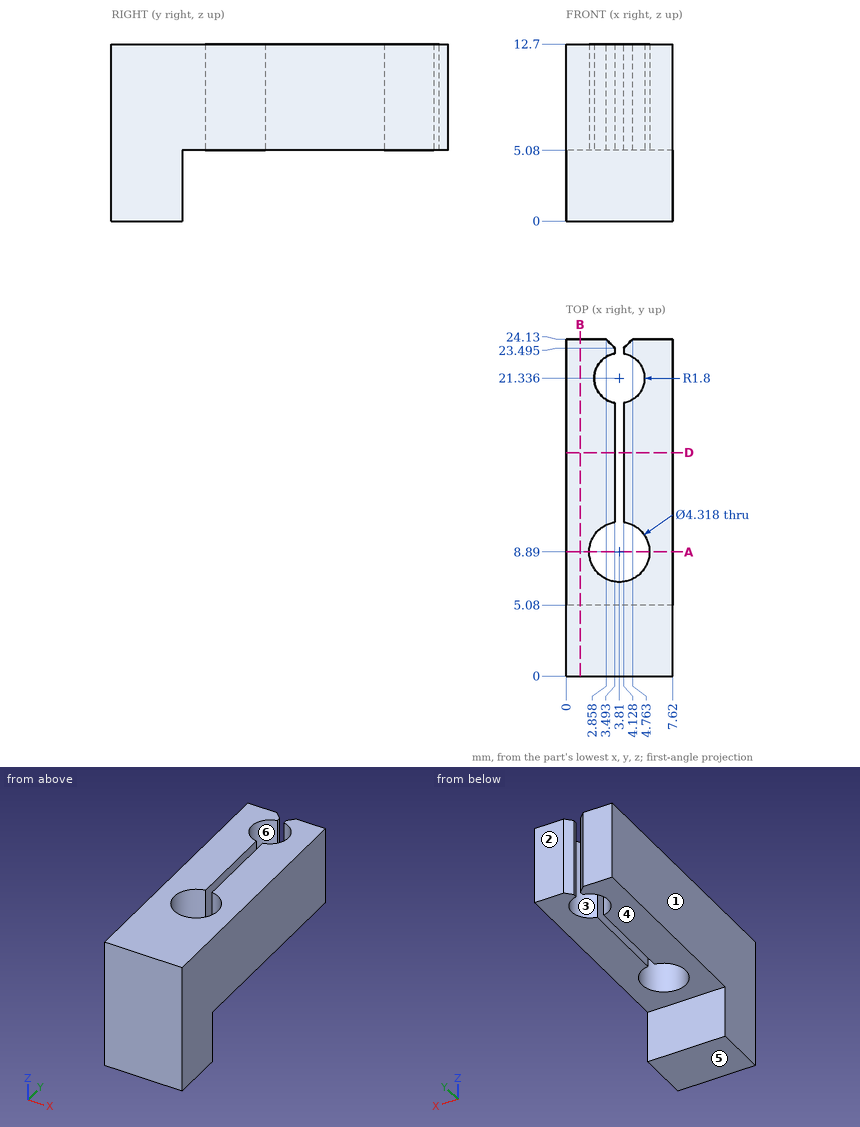
Answer from the drawing. Dimensions are ordinates in mm from the lowest x, y and z of the part. A direction names the side the tool comes from. Coordinates: 2 decimals unless noted, no trailing zeros. Write each loop counter-clockwise with the first axis right and the second up, starting at its lowest first coordinate (ties: lowest second). Pieces come first, ordered by that corner, then holes. Notation, with made-up numbers: (20, 73) - (43, 73) arc R11 cw to (43, 87) - close; hole circle Ø9 at (83, 59). An arc over 180 degrees is marked (long way). One line per question, with ' | ' between items.
Q1. Consider L1, parallel to X at y = 8.89, z = 7; L2, parallel to Y at x = 2.75, z = 10; L3, parallel to X at y = 14, z = 11.75. Determine where each line is inside the solid, lowest interval first. Write a range as [from, to].
Result set:
L1: [0, 1.65], [5.97, 7.62] | L2: [0, 7.01], [10.77, 19.88], [22.79, 24.13] | L3: [0, 3.49], [4.13, 7.62]
Q2. Find section A-A, the plane y = 8.89. Write down the section's boundary in (x, z).
Result set:
outline: (0, 5.08) - (1.65, 5.08) - (1.65, 12.7) - (0, 12.7) - close; (5.97, 5.08) - (7.62, 5.08) - (7.62, 12.7) - (5.97, 12.7) - close
Q3. Find section B-B, the plane x = 1. Write down the section's boundary in (y, z), plus the area to 3 significant figures.
Result set:
outline: (0, 0) - (5.08, 0) - (5.08, 5.08) - (24.13, 5.08) - (24.13, 12.7) - (0, 12.7) - close | area: 210 mm^2
Q4. For the marked faces 4, 5 and 6, determine the directions among +Z, -Z, +X, -X, +Y, -Y from which every point of the face is accessible in a straight line to the end or side of a thin tool.
Result set:
face 4: -Z, +X, -X, +Y | face 5: -Z, +X, -X, +Y, -Y | face 6: +Z, -Z
Q5. Determine the mould class of the marked faces 1, 2 and 3 for opening direction Y: +Y half, -Y half, draft (parallel to the pull), parting line (faces both ways), or undercut.
Result set:
face 1: draft | face 2: +Y half | face 3: undercut
Q6. Find section D-D, the plane y = 16. Write down the section's boundary in (x, z).
Result set:
outline: (0, 5.08) - (3.49, 5.08) - (3.49, 12.7) - (0, 12.7) - close; (4.13, 5.08) - (7.62, 5.08) - (7.62, 12.7) - (4.13, 12.7) - close
Q7. Each of these flat-tipped pins is pushed along its axis until it touches: P1, Ø2, axis at x = 1.5, y = 6.5, coming from the -Z side; P2, Ø2, axis at x = 3, z = 3.5, coming from the -Y side. Where does it stop, or does it pass through?
Result set:
P1: z = 5.08 | P2: y = 0
